Source: CAD feature listing. Evaluate the final solid. Frame: model axes, mm. Face numbers are marked on the shaded views. A direction names the side the tool comes from. Round coordinates to 2 decimals unless told otherwise and drop trailing zeros. Order: outer loops, then holes, each group sorted by start corner. A loop starts at its lowest first (then second) coordinate and runs counter-clockwise, first axis right, second up. Notation, with made-up numbers: M 31.5,77.25 L 58.5,77.25 A23 ccw 58.5,86.25 Z; hole C 58,-22.5 d9. An arc over 180 degrees is marked long. Answer as CSV lines item,"result". Start each with the question number.
Item 1: First-contact query: P1, Ø1.7, axis at x = 1, z = 32, coming from the +Y side. Flat tip, straight axial feed; report the tip coordinate or a pass-through.
Item 2: Line query: line 1 (Z direction, x = 2.65, y = 2.05); line 2 (Z direction, x = 4, y = 1.75); line 3 (Y direction, x = 1.5, z = 10). Output: solid intervals per line, ascending. Write a range as [from, to].
Item 3: Set-up query: the marked faces 1 and 2. Return all of +Z, -Z, +X, -X, +Y, -Y with unobstructed straight access to the full face (end or side cutting, diameter ignored); none if empty.
Item 4: Section query B-B on y = 1.3. Return the cut outline in (x, z).
Item 5: Section query D-D on z = 13. Return the cut outline in (x, y).
Item 6: Pull-direction query (Z, two-part tool) for the marked faces 3, 4 and 5; classes: +Z half, -Z half, draft (parallel to the pull), parting line (faces both ways), or undercut.
Item 7: Section query C-C on x = 2.4. Return the cut outline in (y, z).
Item 8: Section query A-A on z = 32. Return the cut outline in (x, y), plus the area to 3 significant figures.
from build123d import *

# Parameters (mm, degrees)
BOSS_EXTRUDE1_DEPTH = 38.5
FILLET3_R           = 1
FILLET4_R           = 1
CUT_EXTRUDE1_DEPTH  = 2.4
LPATTERN1_COUNT     = 2
LPATTERN1_PITCH     = 12.5
SKETCH3_W           = 5.4
SKETCH3_H           = 8
CUT_EXTRUDE2_DEPTH  = 2.4
FILLET5_R           = 3
FILLET6_R           = 0.35


with BuildPart() as part:
    # Sketch1 → Boss-Extrude1 (new body)
    with BuildSketch(Plane.XY):
        Polygon((0, 0), (3.4, 0), (4.4, 0.663324958), (4.4, 3.263324958), (-1, 3.263324958), (-1, 0.663324958), align=None)
    extrude(amount=BOSS_EXTRUDE1_DEPTH)

    # Fillet3
    fillet3_edges = [part.edges().sort_by_distance(p)[0] for p in [
        (3.4, 0, 19.25),
    ]]
    fillet(fillet3_edges, radius=FILLET3_R)

    # Fillet4
    fillet4_edges = [part.edges().sort_by_distance(p)[0] for p in [
        (0, 0, 19.25),
    ]]
    fillet(fillet4_edges, radius=FILLET4_R)

    # Sketch2 → Cut-Extrude1 (cut)
    with BuildSketch(Plane(origin=(0, 3.263324958, 0), x_dir=(1, 0, 0), z_dir=(0, 1, 0))):
        Polygon((4.4, -9.81), (4.4, -6.48), (1.7, -4.8), (-1, -6.48), (-1, -9.81), (1.7, -11.49), align=None)
    cut_extrude1 = extrude(amount=-CUT_EXTRUDE1_DEPTH, mode=Mode.SUBTRACT)

    # LPattern1: Cut-Extrude1 ×2
    with Locations(*[(0, 0, i * LPATTERN1_PITCH) for i in range(1, LPATTERN1_COUNT)]):
        add(cut_extrude1, mode=Mode.SUBTRACT)

    # Sketch3 → Cut-Extrude2 (cut)
    with BuildSketch(Plane(origin=(0, 3.263324958, 0), x_dir=(1, 0, 0), z_dir=(0, 1, 0))):
        with Locations((1.7, -31.5)):
            Rectangle(SKETCH3_W, SKETCH3_H)
    extrude(amount=-CUT_EXTRUDE2_DEPTH, mode=Mode.SUBTRACT)

    # Fillet5
    # the kernel refuses this fillet: 3 mm, written as the material it adds along each edge
    with BuildSketch(Plane(origin=(4.4, 0.863324958, 27.5), x_dir=(0, 0, 1), z_dir=(-1, 0, 0))) as fillet5_piece_1:
        with BuildLine():
            CenterArc((2.939387691, 3), FILLET5_R, 191.536959033, 78.463040967)
            Line((0, 2.4), (-0.058787754, 2.388))
            ThreePointArc((-0.058787754, 2.388), (-0.06, 1.2), (-0.06, 0))
            Line((-0.06, 0), (0, -0.06))
            Line((0, -0.06), (2.939387691, -0.06))
            Line((2.939387691, -0.06), (2.939387691, 0))
        make_face()
    extrude(amount=5.4)
    with BuildSketch(Plane(origin=(-1, 0.863324958, 35.5), x_dir=(0, 1.0, -1.5483910450100627e-12), z_dir=(1, 0, 0))) as fillet5_piece_2:
        with BuildLine():
            CenterArc((3, -2.939387691), FILLET5_R, 101.536959033, 78.463040967)
            Line((0, -2.939387691), (-0.06, -2.939387691))
            Line((-0.06, -2.939387691), (-0.06, 0))
            Line((-0.06, 0), (0, 0.06))
            ThreePointArc((0, 0.06), (1.2, 0.06), (2.388, 0.058787754))
            Line((2.388, 0.058787754), (2.4, 0))
        make_face()
    extrude(amount=5.4)

    # Fillet6
    fillet6_edges = [part.edges().sort_by_distance(p)[0] for p in [
        (1.7, 2.063324958, 11.49),
        (1.7, 2.063324958, 4.8),
        (1.7, 2.063324958, 23.99),
        (1.7, 2.063324958, 17.3),
    ]]
    fillet(fillet6_edges, radius=FILLET6_R)


solid = part.part
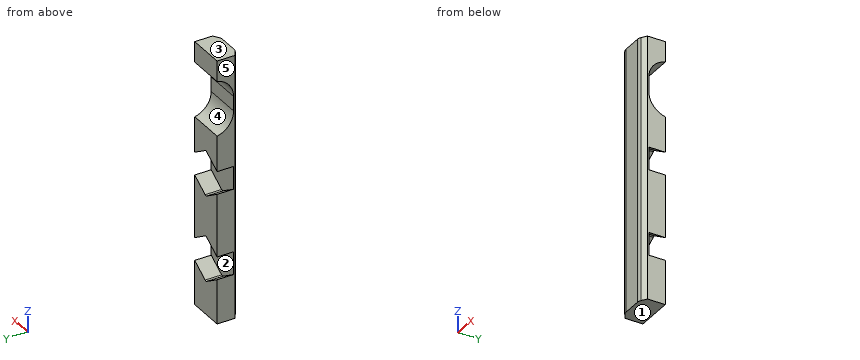
Results:
1,P1,"y = 0.88"
2,line 1,"[0, 5.39], [10.9, 17.89], [23.4, 28.05], [34.95, 38.5]"
2,line 2,"[0, 6.23], [10.06, 18.73], [22.56, 28.31], [34.69, 38.5]"
2,line 3,"[0, 0.86]"
3,face 1,"-Z, +X, -X, +Y, -Y"
3,face 2,"+Y"
4,outline,"M -1,0 L 4.4,0 L 4.4,6.48 L 1.88,4.92 A0.35 cw 1.52,4.92 L -1,6.48 Z; M -1,9.81 L 1.52,11.37 A0.35 cw 1.88,11.37 L 4.4,9.81 L 4.4,18.98 L 1.88,17.42 A0.35 cw 1.52,17.42 L -1,18.98 Z; M -1,22.31 L 1.52,23.87 A0.35 cw 1.88,23.87 L 4.4,22.31 L 4.4,28.88 L -1,28.88 Z; M -1,34.12 L 4.4,34.12 L 4.4,38.5 L -1,38.5 Z"
5,outline,"M -1,0.66 L -0.25,0.17 A1 ccw 0.3,0 L 3.1,0 A1 ccw 3.65,0.17 L 4.4,0.66 L 4.4,3.26 L -1,3.26 Z"
6,face 3,"+Z half"
6,face 4,"undercut"
6,face 5,"draft"
7,outline,"M 0,0 L 3.26,0 L 3.26,5.24 L 0.86,5.24 L 0.86,11.05 L 3.26,11.05 L 3.26,17.74 L 0.86,17.74 L 0.86,23.55 L 3.26,23.55 L 3.26,27.5 A3 cw 0.86,30.44 L 0.86,32.56 A3 cw 3.26,35.5 L 3.26,38.5 L 0,38.5 Z"
8,outline,"M -1,0.66 L -0.25,0.17 A1 ccw 0.3,0 L 3.1,0 A1 ccw 3.65,0.17 L 4.4,0.66 L 4.4,0.86 L -1,0.86 Z"
8,area,"3.98 mm^2"
